from build123d import *

# Parameters (mm, degrees)
BOSS_EXTRUDE1_DEPTH = 17.85
SKETCH5_R           = 1
CUT_EXTRUDE1_DEPTH  = 10
SKETCH6_W           = 34.25
SKETCH6_H           = 9
BOSS_EXTRUDE2_DEPTH = 3


with BuildPart() as part:
    # Sketch4 → Boss-Extrude1 (new body)
    with BuildSketch(Plane(origin=(0, 0, -70.608208955), x_dir=(-1, 0, 0), z_dir=(0, 0, -1))):
        Polygon((-69.066917791, 81.5), (-45.816917791, 81.5), (-45.816917791, 96.6), (-40.316917791, 96.6), (-40.316917791, 78.6), (-74.566917791, 78.6), (-74.566917791, 96.6), (-69.066917791, 96.6), align=None)
    extrude(amount=BOSS_EXTRUDE1_DEPTH)

    # Sketch5 → Cut-Extrude1 (cut)
    with BuildSketch(Plane(origin=(0, 0, -88.458208955), x_dir=(-1, 0, 0), z_dir=(0, 0, -1))):
        with Locations((-43.741917791, 88)):
            Circle(SKETCH5_R)
        with Locations((-71.141917791, 88)):
            Circle(SKETCH5_R)
    extrude(amount=-CUT_EXTRUDE1_DEPTH, mode=Mode.SUBTRACT)

    # Sketch6 → Boss-Extrude2 (add)
    with BuildSketch(Plane(origin=(0, 0, -70.608208955), x_dir=(-1, 0, 0), z_dir=(0, 0, -1))):
        with Locations((-57.441917791, 74.1)):
            Rectangle(SKETCH6_W, SKETCH6_H)
        with BuildLine():
            Line((-68.111940299, 77.5), (-44.896828216, 77.5))
            ThreePointArc((-44.896828216, 77.5), (-42.396828216, 75), (-44.896828216, 72.5))
            Line((-44.896828216, 72.5), (-68.111940299, 72.5))
            ThreePointArc((-68.111940299, 72.5), (-70.611940299, 75), (-68.111940299, 77.5))
        make_face(mode=Mode.SUBTRACT)
    extrude(amount=BOSS_EXTRUDE2_DEPTH)


solid = part.part
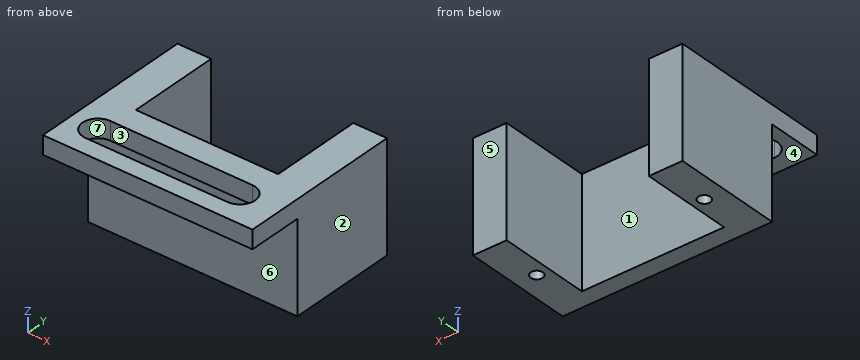
Geometry: final body of the model. Coordinates: model frame, mm. Face numbers are marked on the shaded views. A direction names the side the tool comes from. Coordinates: 2 decimals unless noted, no trailing zeros. Loops run counter-clockwise (first coordinate to the right, second up) from the corner with the lowest first, then second, coordinate; pieces in that order, holes last. Notation, with made-up numbers: (61, -28.5) - (115, -28.5) arc R20 cw to (115, -1.5) - close; hole circle Ø7 at (10.5, 60). An arc over 180 degrees is marked (long way). Put each result on its own line as item: value. Start each with the question number.
Q1. Line query: line 1 (X direction, y = 88, z = -85); line 2 (Y direction, x = 64, z = -71.5); line 3 (X direction, y = 93.25, z = -74.25). Output: solid intervals per line, ascending.
Q2. Cut plane B-B, the plane x = 54.5. Return loops of the section in (y, z), and give its area (3 significant figures).
Q3. Pull-direction query (Y, two-part tool) for the marked faces 5, 6 and 7; classes: released by +Y, released by -Y, zero draft, split by the parting line, or undercut.
Q4. Cut plane A-A, the plane y = 75. Return loops of the section in (x, z), and give its area (3 significant figures).
Q5. Pin query (flat end, axial travel): pin 1 Ø0.6 at (x, y) = (43.5, 88) entering from -Z; pin 2 Ø1.5 at (x, z) = (58.5, -72) entering from +Y. Return the tip coordinate at first contact, or that it passes through.
Q6. Cut plane C-C, the plane z = -81.25. Return loops of the section in (x, y), and give its area (3 significant figures).
Q7. Cut plane D-D, the plane y = 88. Return loops of the section in (x, z).
Q8. Set-up query: the marked faces 1, 2, 3 and 4. Return all of +Z, -Z, +X, -X, +Y, -Y with unobstructed straight access to the full face (end or side cutting, diameter ignored); none if empty.
Filled sheet:
1. line 1: 40.32 to 42.74, 44.74 to 45.82, 69.07 to 70.14, 72.14 to 74.57
1. line 2: 69.6 to 72.5, 77.5 to 81.5
1. line 3: 40.32 to 45.82, 69.07 to 74.57
2. outline: (69.6, -73.61) - (72.5, -73.61) - (72.5, -70.61) - (69.6, -70.61) - close; (77.5, -73.61) - (78.6, -73.61) - (78.6, -88.46) - (81.5, -88.46) - (81.5, -70.61) - (77.5, -70.61) - close
2. area: 63.8 mm²
3. face 5: released by +Y
3. face 6: released by -Y
3. face 7: undercut
4. outline: (40.32, -73.61) - (42.4, -73.61) - (42.4, -70.61) - (40.32, -70.61) - close; (70.61, -73.61) - (74.57, -73.61) - (74.57, -70.61) - (70.61, -70.61) - close
4. area: 18.1 mm²
5. pin 1: z = -78.46
5. pin 2: y = 81.5
6. outline: (40.32, 78.6) - (74.57, 78.6) - (74.57, 96.6) - (69.07, 96.6) - (69.07, 81.5) - (45.82, 81.5) - (45.82, 96.6) - (40.32, 96.6) - close; hole circle Ø2 at (43.74, 88); hole circle Ø2 at (71.14, 88)
6. area: 259 mm²
7. outline: (40.32, -88.46) - (42.74, -88.46) - (42.74, -78.46) - (44.74, -78.46) - (44.74, -88.46) - (45.82, -88.46) - (45.82, -70.61) - (40.32, -70.61) - close; (69.07, -88.46) - (70.14, -88.46) - (70.14, -78.46) - (72.14, -78.46) - (72.14, -88.46) - (74.57, -88.46) - (74.57, -70.61) - (69.07, -70.61) - close
8. face 1: +Z, -Z, +Y
8. face 2: +Z, -Z, +X, +Y, -Y
8. face 3: +Z, -Z
8. face 4: -Z, +X, -X, -Y
